```python
from build123d import *

# Parameters (mm, degrees)
SKETCH2_R          = 5
SKETCH2_R_2        = 7.596705921
CUT_EXTRUDE2_DEPTH = 10


with BuildPart() as part:
    # Sketch1 → Revolve1 (revolve)
    with BuildSketch(Plane.XY):
        with BuildLine():
            Line((-85, 25), (0, 25))
            Line((0, 25), (0, 30))
            Line((0, 30), (-100, 30))
            ThreePointArc((-100, 30), (-115.811388301, 32.565835097), (-130, 40))
            ThreePointArc((-130, 40), (-204.72135955, -22.360679775), (-110, 0))
            ThreePointArc((-110, 0), (-102.67766953, 17.67766953), (-85, 25))
        make_face()
    revolve(axis=Axis((0, 30, 0), (0, -1, 0)))

    # Sketch2 → Cut-Extrude2 (cut)
    with BuildSketch(Plane(origin=(0, 30, 0), x_dir=(1, 0, 0), z_dir=(0, 1, 0))):
        with Locations(Location((0, 75, 0), (0, 0, 180))):
            Circle(SKETCH2_R)
        with Locations(Location((0, 0, 0), (0, 0, 180))):
            Circle(SKETCH2_R_2)
        with Locations(Location((75, 0, 0), (0, 0, 180))):
            Circle(SKETCH2_R)
        with Locations(Location((0, -75, 0), (0, 0, 180))):
            Circle(SKETCH2_R)
        with Locations(Location((-75, 0, 0), (0, 0, 180))):
            Circle(SKETCH2_R)
        with BuildLine():
            Line((-5, 20), (-5, 25))
            ThreePointArc((-5, 25), (0, 30), (5, 25))
            Line((5, 25), (5, 20))
            ThreePointArc((5, 20), (0, 15), (-5, 20))
        make_face()
        with BuildLine():
            Line((20, 5), (25, 5))
            ThreePointArc((25, 5), (30, 0), (25, -5))
            Line((25, -5), (20, -5))
            ThreePointArc((20, -5), (15, 0), (20, 5))
        make_face()
        with BuildLine():
            Line((5, -20), (5, -25))
            ThreePointArc((5, -25), (0, -30), (-5, -25))
            Line((-5, -25), (-5, -20))
            ThreePointArc((-5, -20), (0, -15), (5, -20))
        make_face()
        with BuildLine():
            Line((-20, -5), (-25, -5))
            ThreePointArc((-25, -5), (-30, 0), (-25, 5))
            Line((-25, 5), (-20, 5))
            ThreePointArc((-20, 5), (-15, 0), (-20, -5))
        make_face()
    extrude(amount=-CUT_EXTRUDE2_DEPTH, mode=Mode.SUBTRACT)


solid = part.part
```
Geometry: final body of the model. Coordinates: model frame, mm. A direction names the side the tool comes from. Round coordinates to 2 decimals unless told otherwise and drop trailing zeros. Loops run counter-clockwise (first coordinate to the right, second up) from the corner with the lowest first, then second, coordinate; pieces in that order, holes last. Notation, with made-up numbers: (-19, 17) -> (21, 17) arc R17 ccw to (21, 43) -> close; hole circle Ø11 at (60, 8). An arc over 180 degrees is marked (long way). Write each question's results on one line, items separated by ' | '.
Item 1: Cut plane A-A on z = 0. Return the cut outline in (x, y), and give its area (3 significant figures).
Answers below:
outline: (-130, 40) arc R50 ccw (long way) to (-110, 0) arc R25 cw to (-85, 25) -> (-80, 25) -> (-80, 30) -> (-100, 30) arc R50 cw to start; (-70, 25) -> (-30, 25) -> (-30, 30) -> (-70, 30) -> close; (-15, 25) -> (-7.6, 25) -> (-7.6, 30) -> (-15, 30) -> close; (7.6, 25) -> (15, 25) -> (15, 30) -> (7.6, 30) -> close; (30, 25) -> (70, 25) -> (70, 30) -> (30, 30) -> close; (80, 25) -> (85, 25) arc R25 cw to (110, 0) arc R50 ccw (long way) to (130, 40) arc R50 cw to (100, 30) -> (80, 30) -> close | area: 17,000 mm²
Item 2: Pin query (flat end, axial travel): pin 1 Ø1.5 at (x, y) = (23, 26.5) entering from -Z; pin 2 Ø10 at (y, z) = (-24.5, 165.5) entering from -X; pin 3 Ø2 at (x, y) = (149.5, -29) entering from -Z. Return the tip coordinate at first contact, or that it passes through.
Answers below:
pin 1: stops at z = -201.56 | pin 2: stops at x = -126.53 | pin 3: stops at z = -135.47
Item 3: Cut plane C-C on y = -39.5. Return the cut outline in (x, z).
Answers below:
outline: circle Ø381.31 at (0, 0); hole circle Ø258.69 at (0, 0)
Item 4: Line query: probe 1 along Z at (x, y) = (0, 28.25); probe 2 along Z at (x, y) = (75, 28.95); probe 3 along Z at (x, y) = (15, -40.5). Output: solid intervals per line, ascending. Write a range as [from, to].
Answers below:
probe 1: z = [-201.25, -80], [-70, -30], [-15, -7.6], [7.6, 15], [30, 70], [80, 201.25] | probe 2: z = [-186.23, -5], [5, 186.23] | probe 3: z = [-188.73, -129.81], [129.81, 188.73]
Item 5: Cut plane B-B on x = 0. Return the cut outline in (y, z), and give its area (3 significant figures).
Answers below:
outline: (0, -110) arc R50 ccw (long way) to (40, -130) arc R50 cw to (30, -100) -> (30, -80) -> (25, -80) -> (25, -85) arc R25 cw to start; (0, 110) arc R25 cw to (25, 85) -> (25, 80) -> (30, 80) -> (30, 100) arc R50 cw to (40, 130) arc R50 ccw (long way) to start; (25, -70) -> (30, -70) -> (30, -30) -> (25, -30) -> close; (25, -15) -> (30, -15) -> (30, -7.6) -> (25, -7.6) -> close; (25, 7.6) -> (30, 7.6) -> (30, 15) -> (25, 15) -> close; (25, 30) -> (30, 30) -> (30, 70) -> (25, 70) -> close | area: 17,000 mm²
Item 6: Set-up query: faces 1 (the face through (21, 30, 21)), 2 (the face through (-7.246, 27.535, 2.282)), 3 (the face through (-18, 25, 18)). Return all of +Z, -Z, +X, -X, +Y, -Y with unobstructed straight access to the full face (end or side cutting, diameter ignored); none if empty.
Answers below:
face 1: +Y | face 2: +Y, -Y | face 3: -Y
